Geometry check sheet. Reference: the model listing, model coordinates, mm. Coordinates: 2 decimals unless noted, no trailing zeros. Write each loop counter-clockwise with the first axis right and the second up, starting at its lowest first coordinate (ties: lowest second). Pieces come first, ordered by that corner, then holes. Notation, with made-up numbers: M -14,77 L 43,77 A27 cw 43,103 Z; hole C 61.5,68 d1. An arc over 180 degrees is marked long. Write each question's results on one line, items separated by ' | '.
```python
from build123d import *

# Parameters (mm, degrees)
SKETCH_1_R      = 1
EXTRUDE_1_DEPTH = 10


with BuildPart() as part:
    # 草图1 → 凸台-拉伸1 (new, symmetric)
    with BuildSketch(Plane(origin=(0, 0, 0), x_dir=(1, 0, 0), z_dir=(0, 1, 0))):
        Polygon((2.309401077, 0), (1.154700538, 2), (-1.154700538, 2), (-2.309401077, 0), (-1.154700538, -2), (1.154700538, -2), align=None)
        with Locations(Location((0, 0, 0), (0, 0, 270))):
            Circle(SKETCH_1_R, mode=Mode.SUBTRACT)
    extrude(amount=EXTRUDE_1_DEPTH, both=True)


solid = part.part
```
Q1. Sectioned sample at D-D on x = 1.95. Record the cut outline in (y, z), and give its area (3 significant figures).
Geometry check:
outline: M -10,-0.62 L 10,-0.62 L 10,0.62 L -10,0.62 Z | area: 24.9 mm2
Q2. Scan lines: probe 1 along Z at (x, y) = (0.4, 0.5); probe 2 along X at (y, z) = (-3.75, -0.3); probe 3 along Z at (x, y) = (-0.85, 4). Record each from-to range of solid material in increasing order.
Geometry check:
probe 1: z = -2 to -0.92, 0.92 to 2 | probe 2: x = -2.14 to -0.95, 0.95 to 2.14 | probe 3: z = -2 to -0.53, 0.53 to 2
Q3. Mould release check, pull along X, two halves, no side actions. Record for faces 1 (the cylindrical face through (-1, 0, 0)), 2 (the flat face through (-1.74, 0.14, 0.99)), 3 (the flat face through (-1, -10, -1)): pulls with the +X half, pulls with the -X half, needs draft (parallel to the pull), parting line crosses it, or undercut.
Geometry check:
face 1: undercut | face 2: pulls with the -X half | face 3: needs draft
Q4. Sectioned sample at C-C on y = -8.5. Record the cut outline in (x, z), and give its area (3 significant figures).
Geometry check:
outline: M -2.31,0 L -1.15,-2 L 1.15,-2 L 2.31,0 L 1.15,2 L -1.15,2 Z; hole C 0,0 d2 | area: 10.7 mm2
Q5. Sectioned sample at B-B on z = -0.35. Record the cut outline in (x, y), and give its area (3 significant figures).
Geometry check:
outline: M -2.11,-10 L -0.94,-10 L -0.94,10 L -2.11,10 Z; M 0.94,-10 L 2.11,-10 L 2.11,10 L 0.94,10 Z | area: 46.8 mm2
Q6. Sectioned sample at A-A on x = 0. Record the cut outline in (y, z), and give its area (3 significant figures).
Geometry check:
outline: M -10,-2 L 10,-2 L 10,-1 L -10,-1 Z; M -10,1 L 10,1 L 10,2 L -10,2 Z | area: 40.0 mm2
